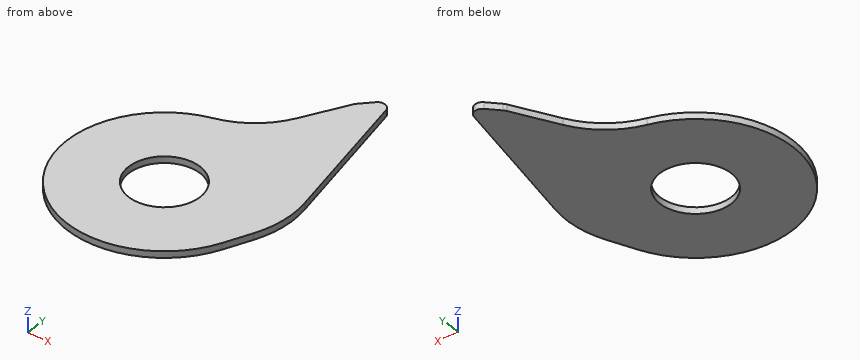
```python
from build123d import *

# Parameters (mm, degrees)
SKETCH1_R      = 27.5
EXTRUDE1_DEPTH = 5


with BuildPart() as part:
    # Sketch1 → Extrude1 (new body)
    with BuildSketch(Plane.XY):
        with BuildLine():
            Line((24.77155023, 103.905583581), (43.516396951, 136.372610482))
            ThreePointArc((43.516396951, 136.372610482), (44.243117586, 137.460224772), (45.105583177, 138.443678294))
            Line((45.105583177, 138.443678294), (53.511867952, 146.849963069))
            ThreePointArc((53.511867952, 146.849963069), (59.558743436, 148.329624086), (63.663355157, 143.649211448))
            Line((63.663355157, 143.649211448), (83.174325272, 32.997001352))
            ThreePointArc((83.174325272, 32.997001352), (83.672108399, 10.183923611), (77.286827824, -11.722981603))
            Line((77.286827824, -11.722981603), (67.973084028, -31.696369631))
            ThreePointArc((67.973084028, -31.696369631), (-58.281283725, -47.204787547), (-16.885768401, 73.074419775))
            ThreePointArc((-16.885768401, 73.074419775), (7.148542121, 84.158707713), (24.77155023, 103.905583581))
        make_face()
        Circle(SKETCH1_R, mode=Mode.SUBTRACT)
    extrude(amount=EXTRUDE1_DEPTH)


solid = part.part
```
CAD build for the part. Positions are in the model's coordinates, mm. Coordinates: 2 decimals unless noted, no trailing zeros. Order: outer loops, then holes, each group sorted by start corner. A loop starts at its lowest first (then second) coordinate and runs counter-clockwise, first axis right, second up. Notation, with made-up numbers: (57.25, 54.25) - (111.25, 54.25) arc R18 cw to (111.25, 72.25) - close; hole circle Ø1 at (-8, -9.5). An arc over 180 degrees is marked (long way). Answer in a Markdown table with one row per item.
1. Drill centre lines: L1, parallel to Y at x = 0, z = 2.6; L2, parallel to Y at x = -4, z = 3.1; L3, parallel to X at y = 20, z = 1.9. Where is each one in solid material? Low to high. Write a range as from..to.
Answer:
| item | result |
|---|---|
| L1 | -75..-27.5, 27.5..79.56 |
| L2 | -74.89..-27.21, 27.21..77.52 |
| L3 | -72.28..-18.87, 18.87..84.31 |
2. Slice it at D-D, the plane x = -36. List the corners of the cut face in (y, z).
Answer:
| item | result |
|---|---|
| outline | (-65.8, 0) - (65.8, 0) - (65.8, 5) - (-65.8, 5) - close |
3. Flat gauge pin, fed straight in: P1, Ø2, axis at x = 43.5, z = 2, coming from the +Y side. Where does the tip first touch, or does it go through?
Answer:
| item | result |
|---|---|
| P1 | y = 137.78 |
4. Slice it at A-A, the plane y = 0. List the corners of the cut face in (x, z).
Answer:
| item | result |
|---|---|
| outline | (-75, 0) - (-27.5, 0) - (-27.5, 5) - (-75, 5) - close; (27.5, 0) - (81.61, 0) - (81.61, 5) - (27.5, 5) - close |
5. Slice it at C-C, the plane z = 2.65. List the corners of the cut face in (x, y), then the cut area to 3 significant figures.
Answer:
| item | result |
|---|---|
| outline | (-16.89, 73.07) arc R75 ccw (long way) to (67.97, -31.7) - (77.29, -11.72) arc R75 ccw to (83.17, 33) - (63.66, 143.65) arc R6 ccw to (53.51, 146.85) - (45.11, 138.44) arc R10 ccw to (43.52, 136.37) - (24.77, 103.91) arc R65 cw to start; hole circle Ø55 at (0, 0) |
| area | 20,100 mm² |
6. Slice it at B-B, the plane x = -7. List the corners of the cut face in (y, z).
Answer:
| item | result |
|---|---|
| outline | (-74.67, 0) - (-26.59, 0) - (-26.59, 5) - (-74.67, 5) - close; (26.59, 0) - (76.21, 0) - (76.21, 5) - (26.59, 5) - close |
